The model under review builds one solid part; all positions refer to its coordinate system, in mm. Face numbers are marked on the shaded views. Coordinates: 2 decimals unless noted, no trailing zeros. Order: outer loops, then holes, each group sorted by start corner. A loop starts at its lowest first (then second) coordinate and runs counter-clockwise, first axis right, second up. Notation, with made-up numbers: (19, 79.5) - (25, 79.5) arc R31 cw to (25, 114.5) - close; hole circle Ø9 at (69.25, 78). An arc over 180 degrees is marked (long way). Answer in a Markdown table with one row per item.
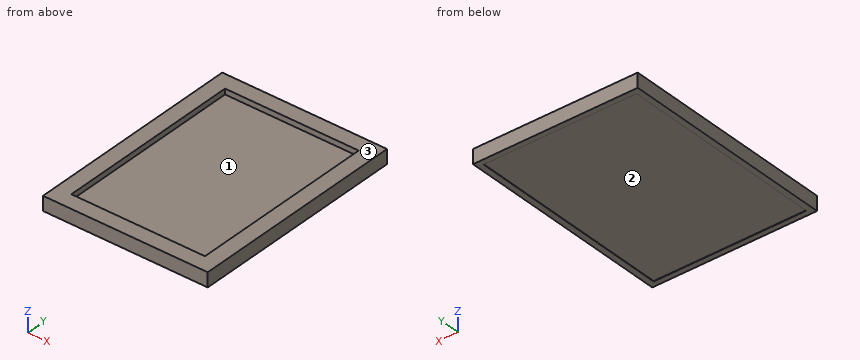
Solid Edge part; units mm, degrees
sketch "Sketch1" plane through (0, 0, 0) normal (0, 0, 1) x (1, 0, 0)
  line L0 (92.5, 122.5) -> (-92.5, 122.5)
  line L1 (-92.5, 122.5) -> (-92.5, -122.5)
  line L2 (-92.5, -122.5) -> (92.5, -122.5)
  line L3 (92.5, -122.5) -> (92.5, 122.5)
extrude "Protrusion1" add sketch "Sketch1" along normal blind 16
sketch "Sketch2" plane through (0, 0, 0) normal (0, 0, -1) x (-1, 0, 0)
  line L0 (-85.75, 116.25) -> (-85.75, -116.25)
  line L1 (-85.75, -116.25) -> (85.75, -116.25)
  line L2 (85.75, -116.25) -> (85.75, 116.25)
  line L3 (85.75, 116.25) -> (-85.75, 116.25)
extrude "Wycięcie_1" cut sketch "Sketch2" along normal mid plane 1
sketch "Sketch3" plane through (0, 0, 16) normal (0, 0, 1) x (1, 0, 0)
  line L0 (75, 105) -> (-75, 105)
  line L1 (-75, 105) -> (-75, -105)
  line L2 (-75, -105) -> (75, -105)
  line L3 (75, -105) -> (75, 105)
extrude "Wycięcie_2" cut sketch "Sketch3" along normal mid plane 12.4
properties material "Aluminium, 1060"
Item 1: Clearance check with flat-ended pins moving along their axes: pin 1 Ø10 at (x, y) = (-58, 88.5) entering from +Z; pin 2 Ø12 at (x, y) = (-7.5, -27) entering from -Z. State where each tip first meets the part, or that it passes through.
Check values:
| item | result |
|---|---|
| pin 1 | z = 9.8 |
| pin 2 | z = 0.5 |
Item 2: To check wall thickness, follow line 1 (X direction, y = 91, z = 12.5); line 2 (Z direction, x = -24, y = -62); line 3 (Z direction, x = 42, y = 112). State the ranges of each line that lie inside material, in increasing order. Write a range as from..to.
Check values:
| item | result |
|---|---|
| line 1 | -92.5..-75, 75..92.5 |
| line 2 | 0.5..9.8 |
| line 3 | 0.5..16 |
Item 3: We need section C-C, the plane x = 13.5. Write out the cut boundary in (y, z), then the cut area to 3 significant figures.
Check values:
| item | result |
|---|---|
| outline | (-122.5, 0) - (-116.25, 0) - (-116.25, 0.5) - (116.25, 0.5) - (116.25, 0) - (122.5, 0) - (122.5, 16) - (105, 16) - (105, 9.8) - (-105, 9.8) - (-105, 16) - (-122.5, 16) - close |
| area | 2,500 mm^2 |
Item 4: We need section A-A, the plane y = 77. Write out the cut boundary in (x, z), then the cut area to 3 significant figures.
Check values:
| item | result |
|---|---|
| outline | (-92.5, 0) - (-85.75, 0) - (-85.75, 0.5) - (85.75, 0.5) - (85.75, 0) - (92.5, 0) - (92.5, 16) - (75, 16) - (75, 9.8) - (-75, 9.8) - (-75, 16) - (-92.5, 16) - close |
| area | 1,940 mm^2 |
Item 5: Mouldability with a two-part tool opening along Y and no side actions: class the marked faces 1, 2 and 3 as +Y half, -Y half, draft (parallel to the pull), parting line (faces both ways), or undercut.
Check values:
| item | result |
|---|---|
| face 1 | undercut |
| face 2 | undercut |
| face 3 | draft |
Item 6: We need section B-B, the plane z = 13.5. Write out the cut boundary in (x, y), then the cut area to 3 significant figures.
Check values:
| item | result |
|---|---|
| outline | (-92.5, -122.5) - (92.5, -122.5) - (92.5, 122.5) - (-92.5, 122.5) - close; hole (-75, -105) - (75, -105) - (75, 105) - (-75, 105) - close |
| area | 13,800 mm^2 |
